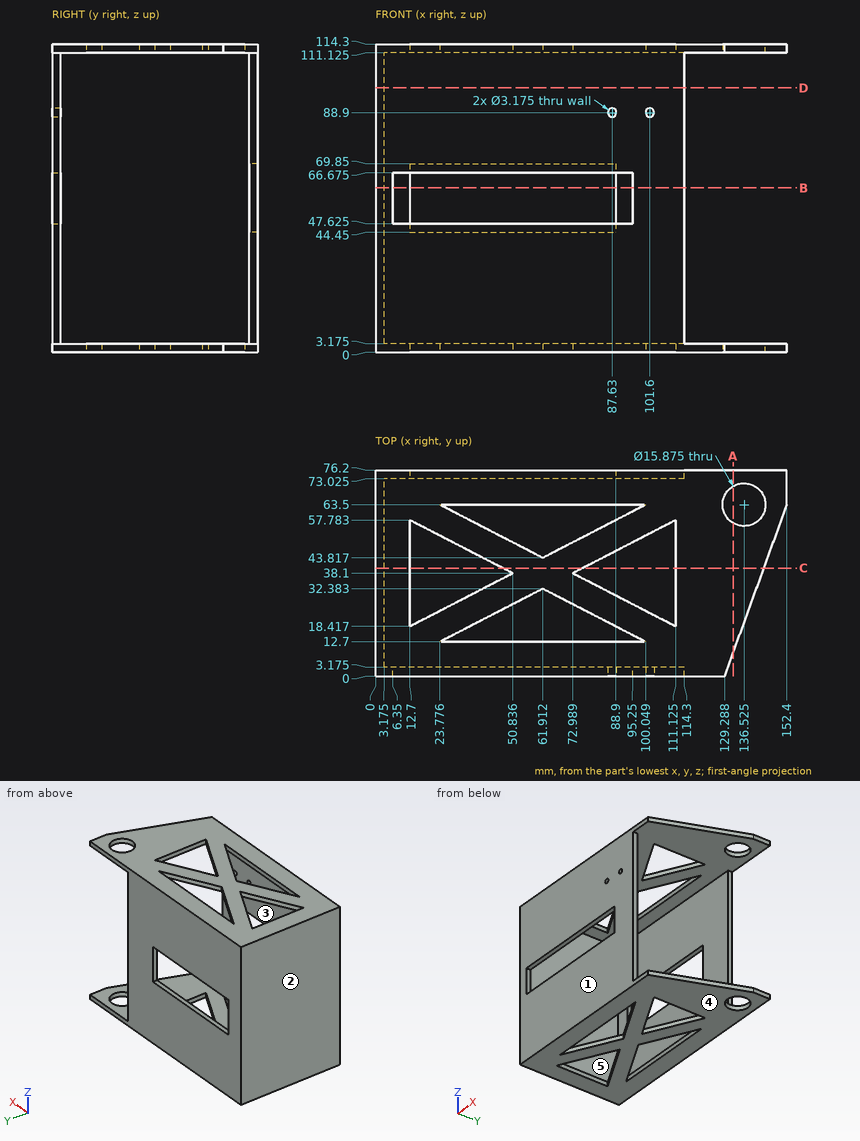
Job drawing, mm, ordinate dimensions from the low corner. One solid piece. A direction names the side the tool comes from. Round coordinates to 2 decimals unless told otherwise and drop trailing zeros. Order: outer loops, then holes, each group sorted by start corner. A loop starts at its lowest first (then second) coordinate and runs counter-clockwise, first axis right, second up. Notation, with made-up numbers: (83, 80.25) - (99, 80.25) arc R13 ccw to (99, 95.25) - close; hole circle Ø2 at (-35.75, 1.5). An arc over 180 degrees is marked (long way). Use CSV: the item, a comma, the result in double quotes. Start each with the question number.
1) Tool access for the marked faces 4 and 5: list every direction of +Z, -Z, +X, -X, +Y, -Y with a clear straight run to the whole face (end or side of a thin tool).
2) Two-plate mould, pull along Y, no slides. Class the marked faces 1, 2 and 3: pulls with the +Y half, pulls with the -Y half, needs draft (parallel to the pull), parting line crosses it, or undercut.
3) Saw through at B-B (z = 61). Count the separate pieces of the cut face and the enclosed holes in it.
4) Pin check, flat tips, straight feed: pin 1 Ø3 at (y, z) = (36, 69) entering from +X (1 decimal); pin 2 Ø1.6 at (y, z) = (74, 61.5) entering from +X; pin 3 Ø3.5 at (y, z) = (39.5, 113) entering from +X. Stop position of each tip, or through.
5) Saw through at C-C (y = 40). List the corners of the cut face in (x, z) (1 decimal).
6) Saw through at D-D (z = 98). List the corners of the cut face in (x, y) (1 decimal).
7) Wall check: L1, parallel to X at y = 0.7, z = 88.9; L2, parallel to Y at x = 47, z = 7.5 (1 decimal); L3, parallel to Z at x = 140, y = 47 (1 decimal). Give the ranges that are in metal, low to high. Write a range as [from, to].
8) Saw through at A-A (x = 132.5). List the corners of the cut face in (y, z) (1 decimal).
Values follow:
1,face 4,"-Z, +X, -X, +Y, -Y"
1,face 5,"+X"
2,face 1,"pulls with the -Y half"
2,face 2,"needs draft"
2,face 3,"undercut"
3,separate pieces,"3"
3,enclosed holes,"0"
4,pin 1,"stops at x = 3.2"
4,pin 2,"stops at x = 114.3"
4,pin 3,"stops at x = 144.3"
5,outline,"(0, 0) - (12.7, 0) - (12.7, 3.2) - (3.2, 3.2) - (3.2, 111.1) - (12.7, 111.1) - (12.7, 114.3) - (0, 114.3) - close; (47.2, 0) - (76.7, 0) - (76.7, 3.2) - (47.2, 3.2) - close; (47.2, 111.1) - (76.7, 111.1) - (76.7, 114.3) - (47.2, 114.3) - close; (111.1, 0) - (143.8, 0) - (143.8, 3.2) - (111.1, 3.2) - close; (111.1, 111.1) - (143.8, 111.1) - (143.8, 114.3) - (111.1, 114.3) - close"
6,outline,"(0, 0) - (114.3, 0) - (114.3, 3.2) - (3.2, 3.2) - (3.2, 73) - (114.3, 73) - (114.3, 76.2) - (0, 76.2) - close"
7,L1,"x = [0, 86.04], [89.22, 100.01], [103.19, 114.3]"
7,L2,"y = [0, 3.2], [73, 76.2]"
7,L3,"z = [0, 3.2], [111.1, 114.3]"
8,outline,"(8.8, 0) - (56.7, 0) - (56.7, 3.2) - (8.8, 3.2) - close; (8.8, 111.1) - (56.7, 111.1) - (56.7, 114.3) - (8.8, 114.3) - close; (70.3, 0) - (76.2, 0) - (76.2, 3.2) - (70.3, 3.2) - close; (70.3, 111.1) - (76.2, 111.1) - (76.2, 114.3) - (70.3, 114.3) - close"
